from build123d import *

# Parameters (mm, degrees)
SKETCH1_W           = 25.4
SKETCH1_H           = 12.7
BOSS_EXTRUDE1_DEPTH = 12.7
SKETCH2_R           = 1.5
CUT_EXTRUDE1_DEPTH  = 5.08
SKETCH4_W           = 11.43
SKETCH4_H           = 5.08
CUT_EXTRUDE3_DEPTH  = 27.432
SKETCH6_W           = 5.588
SKETCH6_H           = 2.54
CUT_EXTRUDE5_DEPTH  = 9.652
SKETCH7_W           = 2.54
SKETCH7_H           = 1.27
CUT_EXTRUDE6_DEPTH  = 26.924


with BuildPart() as part:
    # Sketch1 → Boss-Extrude1 (new body)
    with BuildSketch(Plane.XY):
        Rectangle(SKETCH1_W, SKETCH1_H)
    extrude(amount=BOSS_EXTRUDE1_DEPTH)

    # Sketch2 → Cut-Extrude1 (cut)
    with BuildSketch(Plane(origin=(0, 6.35, 0), x_dir=(1, 0, 0), z_dir=(0, 1, 0))):
        with Locations(Location((-10.16, -2.54, 0), (0, 0, 270))):
            Circle(SKETCH2_R)
        with Locations(Location((10.16, -2.54, 0), (0, 0, 270))):
            Circle(SKETCH2_R)
    extrude(amount=-CUT_EXTRUDE1_DEPTH, mode=Mode.SUBTRACT)

    # Sketch4 → Cut-Extrude3 (cut)
    with BuildSketch(Plane(origin=(12.7, 0, 0), x_dir=(0, 0, -1), z_dir=(1, 0, 0))):
        with Locations((-6.985, -2.54)):
            Rectangle(SKETCH4_W, SKETCH4_H)
    extrude(amount=-CUT_EXTRUDE3_DEPTH, mode=Mode.SUBTRACT)

    # Sketch6 → Cut-Extrude5 (cut)
    with BuildSketch(Plane(origin=(0, 6.35, 0), x_dir=(1, 0, 0), z_dir=(0, 1, 0))):
        with Locations((0, -2.54)):
            Rectangle(SKETCH6_W, SKETCH6_H)
    extrude(amount=-CUT_EXTRUDE5_DEPTH, mode=Mode.SUBTRACT)

    # Sketch7 → Cut-Extrude6 (cut)
    with BuildSketch(Plane(origin=(12.7, 0, 0), x_dir=(0, 0, -1), z_dir=(1, 0, 0))):
        with Locations((-6.35, 0.635)):
            Rectangle(SKETCH7_W, SKETCH7_H)
    extrude(amount=-CUT_EXTRUDE6_DEPTH, mode=Mode.SUBTRACT)


solid = part.part
Geometry check sheet. Reference: the model listing, model coordinates, mm. A direction names the side the tool comes from. Give positions to 0.01 mm unless a question says otherwise; leave off trailing zeros. Order: outer loops, then holes, each group sorted by start corner. A loop starts at its lowest first (then second) coordinate and runs counter-clockwise, first axis right, second up. Notation, with made-up numbers: (2, 67) - (28, 67) arc R16 ccw to (28, 93) - close; hole circle Ø10 at (37.5, -7.75). An arc over 180 degrees is marked (long way). Use one line per item in the form item = value.
1) Sectioned sample at C-C (x = 1). Record the boundary of the cut face in (y, z).
Working result:
outline = (-6.35, 0) - (6.35, 0) - (6.35, 1.27) - (-5.08, 1.27) - (-5.08, 12.7) - (-6.35, 12.7) - close; (0, 3.81) - (6.35, 3.81) - (6.35, 12.7) - (0, 12.7) - (0, 7.62) - (1.27, 7.62) - (1.27, 5.08) - (0, 5.08) - close
2) Sectioned sample at D-D (x = 10.16). Record the boundary of the cut face in (y, z).
Working result:
outline = (-6.35, 0) - (6.35, 0) - (6.35, 1.04) - (1.27, 1.04) - (1.27, 4.04) - (6.35, 4.04) - (6.35, 12.7) - (0, 12.7) - (0, 7.62) - (1.27, 7.62) - (1.27, 5.08) - (0, 5.08) - (0, 1.27) - (-5.08, 1.27) - (-5.08, 12.7) - (-6.35, 12.7) - close
3) Access from +Z, -Z, +X, -X, +Y, -Y to the whole of each face (thin tool, end or side, straight path). Record for faces 4 (the face through (12.7, 1.3, 4.8)), 5 (the face through (-2.794, 3, 3)), 6 (the face through (0, 0, 4)), 7 (the face through (0, -2, 1.27)), 8 (the face through (0, 1, 7.62)).
Working result:
face_4 = +Z, -Z, +X, +Y, -Y
face_5 = +Y
face_6 = +Z, +X, -X
face_7 = none
face_8 = +X, -X
4) Material ranges on probe 1 along X at (y, z) = (5.5, 2.5); probe 2 along Y at (x, z) = (-8.25, 10.5); probe 3 along Z at (x, y) = (6.75, 1), recorded low to high. Write a range as from..to.
Working result:
probe_1 = -12.7..-11.66, -8.66..-2.79, 2.79..8.66, 11.66..12.7
probe_2 = -6.35..-5.08, 0..6.35
probe_3 = 0..5.08, 7.62..12.7
5) Sectioned sample at B-B (z = 4.75). Record the boundary of the cut face in (x, y), and give its area (3 significant figures).
Working result:
outline = (-12.7, -6.35) - (12.7, -6.35) - (12.7, -5.08) - (-12.7, -5.08) - close; (-12.7, 0) - (12.7, 0) - (12.7, 6.35) - (-12.7, 6.35) - close
area = 194 mm^2
6) Draft check along X on faces 1 (the face through (9.585, 3.846, 3.926)), 2 (the face through (0, -5.08, 7)), 3 (the face through (-12.7, 1.3, 4.8)). Enter one of: released by +X, released by -X, zero draft, split by the parting line, or undercut.
Working result:
face_1 = undercut
face_2 = zero draft
face_3 = released by -X
7) Depth check by flat-ended pin: pin 1 Ø3.5 at (x, z) = (-10, 2) entering from +Y; pin 2 Ø3 at (y, z) = (-2.5, 3) entering from -X. Enter the tip coordinate at first touch or a pass-through.
Working result:
pin_1 = 6.35
pin_2 = through
8) Sectioned sample at A-A (z = 2.54). Record the boundary of the cut face in (x, y).
Working result:
outline = (-12.7, -6.35) - (12.7, -6.35) - (12.7, -5.08) - (-12.7, -5.08) - close; (-12.7, 0) - (-2.79, 0) - (-2.79, 6.35) - (-8.66, 6.35) - (-8.66, 1.27) - (-11.66, 1.27) - (-11.66, 6.35) - (-12.7, 6.35) - close; (2.79, 0) - (12.7, 0) - (12.7, 6.35) - (11.66, 6.35) - (11.66, 1.27) - (8.66, 1.27) - (8.66, 6.35) - (2.79, 6.35) - close
